Part model, mm, in its own coordinate system. Face numbers are marked on the shaded views. Round coordinates to 2 decimals unless told otherwise and drop trailing zeros. Loops run counter-clockwise (first coordinate to the right, second up) from the corner with the lowest first, then second, coordinate; pieces in that order, holes last. Notation, with made-up numbers: M 2.5,29.5 L 22.5,29.5 A12 ccw 22.5,44.5 Z; hole C 44.25,-30 d8. An arc over 180 degrees is marked long. Put each result on its own line as item: value. Start each with the question number.
```python
from build123d import *

# Parameters (mm, degrees)
F1_DEPTH = 31.75
F3_D     = 14.2875
F4_R     = 12.7


# Not quite as in the source:
# - a length typed as a fraction of an inch, garbled in the dataset ("3 / 203.2 mm" for 3/8 in), is restored


with BuildPart() as f1:
    # F0 (on Front) → F1 (new body)
    with BuildSketch(Plane.XZ):
        Polygon((0, 66.675), (0, 0), (139.192, 0), (139.192, 66.675), (113.792, 66.675), (104.521, 31.115), (34.671, 31.115), (25.4, 66.675), align=None)
    extrude(amount=F1_DEPTH)

    # F3 (through all)
    with Locations(Plane.YZ.offset(139.192)):
        with Locations((-15.875, 44.45)):
            Hole(F3_D / 2)

    # F4
    f4_edges = [f1.edges().sort_by_distance(p)[0] for p in [
        (69.596, -31.75, 31.115),
    ]]
    fillet(f4_edges, radius=F4_R)


solid = f1.part
```
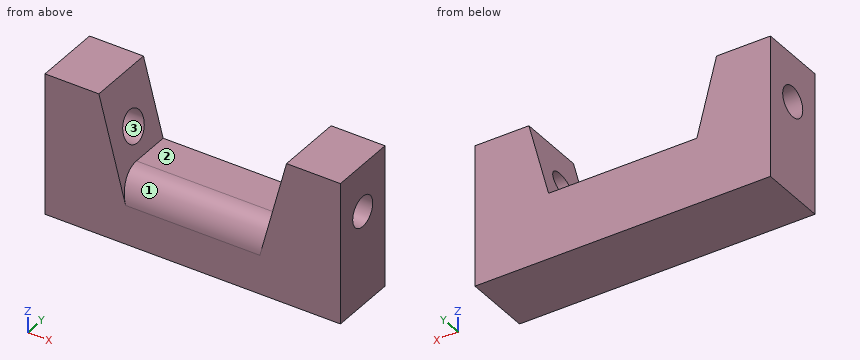
1. Drop a flat-ended pin along its axis: pin 1 (9.5 mm diameter, centred on x = 70, y = -5, fed in from +Z) (3 decimals). Give the stop position or say it passes through.
2. Cut at A-A, the plane z = 44.45. Give the cut face in (x, y).
3. Wall check: L1, parallel to Y at x = 6, z = 45; L2, parallel to Y at x = 18, z = 44.45; L3, parallel to Z at x = 35.5, y = -15 (3 decimals). Give the ranges that are in metal, low to high.
4. Mould opens along Y. For the marked faces 1, 2 and 3 say: released by +Y, released by -Y, zero draft, split by the parting line, or undercut.
5. Cut at C-C, the plane y = -13.5. Give the cut face in (x, z) (3 decimals).
6. Cut at B-B, the plane z = 54. Give the cut face in (x, y).
7. Cut at D-D, the plane y = -26. Give the cut face in (x, z) (3 decimals).
Results list:
1. pin 1: stops at z = 31.115
2. outline: M 0,-31.75 L 31.19,-31.75 L 31.19,-23.02 L 0,-23.02 Z; M 0,-8.73 L 31.19,-8.73 L 31.19,0 L 0,0 Z; M 108,-31.75 L 139.19,-31.75 L 139.19,-23.02 L 108,-23.02 Z; M 108,-8.73 L 139.19,-8.73 L 139.19,0 L 108,0 Z
3. L1: y = -31.75 to -23, -8.75 to 0
3. L2: y = -31.75 to -23.02, -8.73 to 0
3. L3: z = 0 to 31.115
4. face 1: released by -Y
4. face 2: zero draft
4. face 3: undercut
5. outline: M 0,0 L 139.192,0 L 139.192,37.713 L 106.241,37.713 L 104.521,31.115 L 34.671,31.115 L 32.951,37.713 L 0,37.713 Z; M 0,51.187 L 29.438,51.187 L 25.4,66.675 L 0,66.675 Z; M 109.754,51.187 L 139.192,51.187 L 139.192,66.675 L 113.792,66.675 Z
6. outline: M 0,-31.75 L 28.7,-31.75 L 28.7,0 L 0,0 Z; M 110.49,-31.75 L 139.19,-31.75 L 139.19,0 L 110.49,0 Z
7. outline: M 0,0 L 139.192,0 L 139.192,66.675 L 113.792,66.675 L 103.981,29.045 L 35.211,29.045 L 25.4,66.675 L 0,66.675 Z
